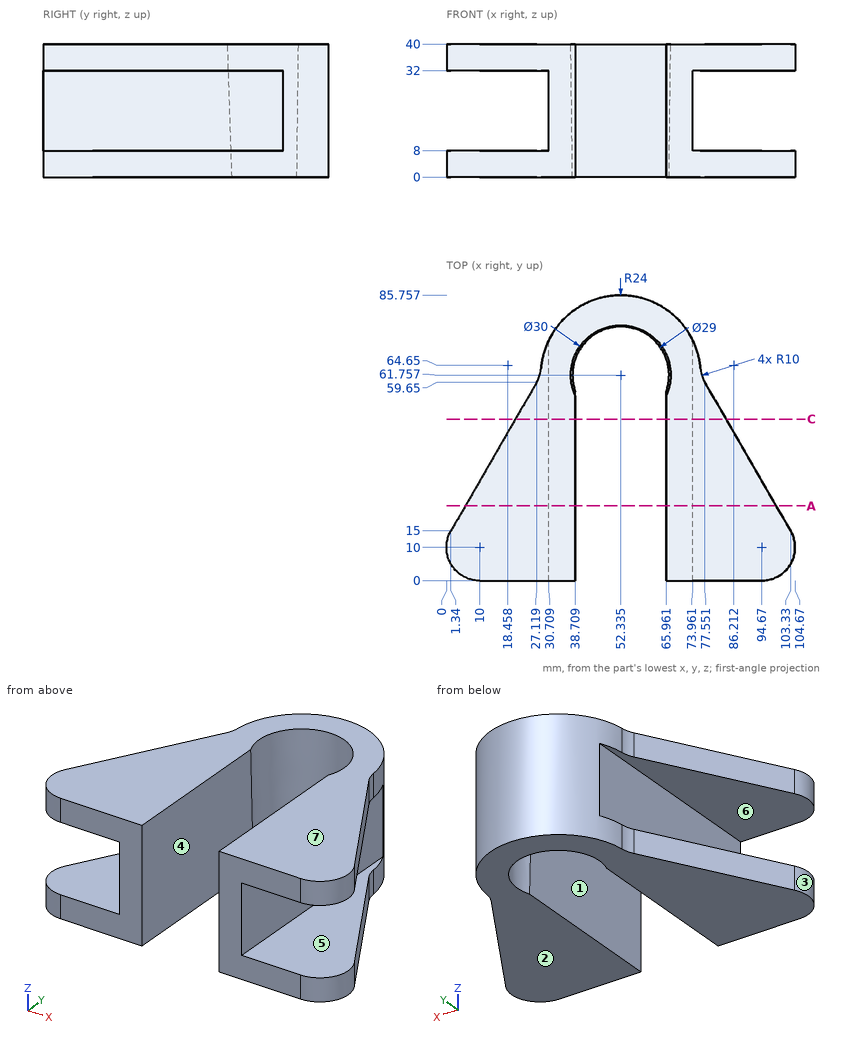
Verification items for this drawing (mm, ordinates from the low corner). A direction names the side the tool comes from. Round coordinates to 2 decimals unless told otherwise and drop trailing zeros. Order: outer loops, then holes, each group sorted by start corner. A loop starts at its lowest first (then second) coordinate and runs counter-clockwise, first axis right, second up. Notation, with made-up numbers: M 71,28 L 111,28 A18 ccw 111,43 Z; hole C 38,-3 d11. An arc over 180 degrees is marked long. Answer in a Markdown table with one row per item. Add a question column.
Item 1: Depth check by flat-ended pin: pin 1 Ø1 at (y, z) = (67, 24.5) entering from -X; pin 2 Ø12 at (x, z) = (65, 5.5) entering from +Y. Enter the tip coordinate at first touch or a pass-through.
Item 2: Sectioned sample at C-C, the plane y = 48.5. Enter the section's corners in (x, z).
Item 3: Sectioned sample at A-A, the plane y = 22.5. Enter the section's corners in (x, z), plus the area to 3 significant figures.
Item 4: Draft check along X on the marked faces 1, 2, 3 and 4. Enter one of: released by +X, released by -X, zero draft, split by the parting line, or undercut.
Item 5: Set-up check for the marked faces 5, 6 and 7: record each of +Z, -Z, +X, -X, +Y, -Y from which the full face is reachable in a straight line by a thin tool's end or side.
Item 6: Material ranges on L1, parallel to X at y = 48.5, z = 31; L2, parallel to Z at x = 77.5, y = 43; L3, parallel to X at y = 31.5, z = 2 (1 decimal), recorded low to high. Write a range as [from, to].
Filled in:
| question | item | result |
|---|---|---|
| 1 | pin 1 | stops at x = 30.71 |
| 1 | pin 2 | stops at y = 84.81 |
| 2 | outline | M 20.68,0 L 38.71,0 L 38.71,40 L 20.68,40 L 20.68,32 L 30.71,32 L 30.71,8 L 20.68,8 Z; M 65.96,0 L 83.99,0 L 83.99,8 L 73.96,8 L 73.96,32 L 83.99,32 L 83.99,40 L 65.96,40 Z |
| 3 | outline | M 5.67,0 L 38.71,0 L 38.71,40 L 5.67,40 L 5.67,32 L 30.71,32 L 30.71,8 L 5.67,8 Z; M 65.96,0 L 99,0 L 99,8 L 73.96,8 L 73.96,32 L 99,32 L 99,40 L 65.96,40 Z |
| 3 | area | 1,440 mm² |
| 4 | face 1 | undercut |
| 4 | face 2 | zero draft |
| 4 | face 3 | released by -X |
| 4 | face 4 | undercut |
| 5 | face 5 | +X, +Y, -Y |
| 5 | face 6 | -X, +Y, -Y |
| 5 | face 7 | +Z, +X, -X, +Y, -Y |
| 6 | L1 | x = [30.71, 38.71], [65.96, 73.96] |
| 6 | L2 | z = [0, 8], [32, 40] |
| 6 | L3 | x = [10.9, 38.7], [66, 93.8] |
